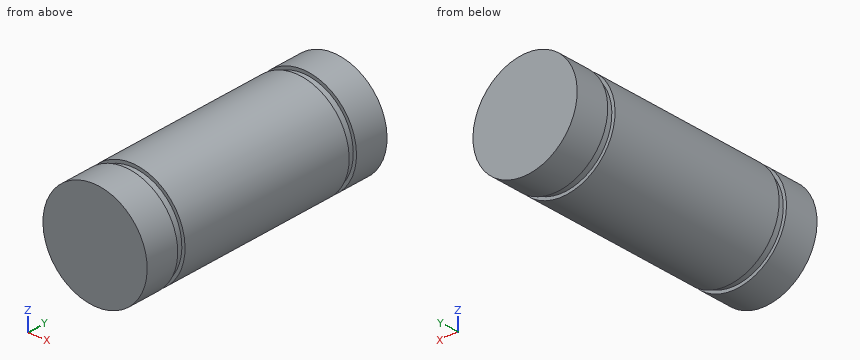
```python
from build123d import *

# Parameters (mm, degrees)
BOSS_EXTRUDE1_DEPTH      = 8.255
BOSS_EXTRUDE1_DEPTH_BACK = 8.255
SKETCH1_R                = 4.7625
SKETCH2_R                = 4.7625
BOSS_EXTRUDE2_DEPTH      = 3.81
BOSS_EXTRUDE3_START      = 3.81
SKETCH3_R                = 4.7625
BOSS_EXTRUDE3_DEPTH      = 3.81
SKETCH4_R                = 5.08
CUT_EXTRUDE1_DEPTH       = 0.7366
SKETCH5_R                = 5.08
CUT_EXTRUDE2_DEPTH       = 0.7366
SKETCH6_R                = 4.4704
BOSS_EXTRUDE4_DEPTH      = 0.7366
SKETCH7_R                = 4.4704
BOSS_EXTRUDE5_DEPTH      = 0.7366


with BuildPart() as part:
    # Sketch1 → Boss-Extrude1 (new, two sides: drawn at the far end of the back side and taken through both)
    with BuildSketch(Plane(origin=(0, 0, 0), x_dir=(1, 0, 0), z_dir=(0, 1, 0)).offset(-BOSS_EXTRUDE1_DEPTH_BACK)):
        with Locations(Location((0, 0, 0), (0, 0, 270))):
            Circle(SKETCH1_R)
    extrude(amount=BOSS_EXTRUDE1_DEPTH + BOSS_EXTRUDE1_DEPTH_BACK)

    # Sketch2 → Boss-Extrude2 (add)
    with BuildSketch(Plane(origin=(0, 8.255, 0), x_dir=(1, 0, 0), z_dir=(0, 1, 0))):
        with Locations(Location((0, 0, 0), (0, 0, 270))):
            Circle(SKETCH2_R)
    extrude(amount=BOSS_EXTRUDE2_DEPTH)

    # Sketch3 → Boss-Extrude3 (add)
    with BuildSketch(Plane(origin=(0, -8.255, 0), x_dir=(-1, 0, 0), z_dir=(0, -1, 0)).offset(BOSS_EXTRUDE3_START)):
        with Locations(Location((0, 0, 0), (0, 0, 90))):
            Circle(SKETCH3_R)
    extrude(amount=-BOSS_EXTRUDE3_DEPTH)

    # Sketch4 → Cut-Extrude1 (cut)
    with BuildSketch(Plane(origin=(0, -8.9916, 0), x_dir=(-1, 0, 0), z_dir=(0, -1, 0))):
        Circle(SKETCH4_R)
    extrude(amount=-CUT_EXTRUDE1_DEPTH, mode=Mode.SUBTRACT)


with BuildPart() as cut_extrude1_piece_1:
    # of the separate pieces the step leaves, piece 1, a body of its own (cut_extrude1_pieces)
    add(part.part.solids().sort_by_distance((0, 12.065, 4.7625))[0])

    # Sketch5 → Cut-Extrude2 (cut)
    with BuildSketch(Plane(origin=(0, 8.9916, 0), x_dir=(1, 0, 0), z_dir=(0, 1, 0))):
        Circle(SKETCH5_R)
    extrude(amount=-CUT_EXTRUDE2_DEPTH, mode=Mode.SUBTRACT)


with BuildPart() as cut_extrude1_piece_2:
    # of the separate pieces the step leaves, piece 2, a body of its own (cut_extrude1_pieces)
    add(part.part.solids().sort_by_distance((0, -12.065, -4.7625))[0])



with BuildPart() as cut_extrude2_piece_1:
    # of the separate pieces the step leaves, piece 1, a body of its own (cut_extrude2_pieces)
    add(cut_extrude1_piece_1.part.solids().sort_by_distance((0, 8.255, 4.7625))[0])


with BuildPart() as cut_extrude2_piece_2:
    # of the separate pieces the step leaves, piece 2, a body of its own (cut_extrude2_pieces)
    add(cut_extrude1_piece_1.part.solids().sort_by_distance((0, 12.065, 4.7625))[0])


with BuildPart() as cut_extrude1_piece_2_1:
    add(cut_extrude1_piece_2.part)

    add(cut_extrude2_piece_1.part)  # Boss-Extrude4 merges Cut-Extrude2 piece 1
    # Sketch6 → Boss-Extrude4 (add)
    with BuildSketch(Plane(origin=(0, -8.9916, 0), x_dir=(1, 0, 0), z_dir=(0, 1, 0))):
        with Locations(Location((0, 0, 0), (0, 0, 90))):
            Circle(SKETCH6_R)
    extrude(amount=BOSS_EXTRUDE4_DEPTH)


    add(cut_extrude2_piece_2.part)  # Boss-Extrude5 merges Cut-Extrude2 piece 2
    # Sketch7 → Boss-Extrude5 (add)
    with BuildSketch(Plane(origin=(0, 8.255, 0), x_dir=(1, 0, 0), z_dir=(0, 1, 0))):
        with Locations(Location((0, 0, 0), (0, 0, 270))):
            Circle(SKETCH7_R)
    extrude(amount=BOSS_EXTRUDE5_DEPTH)


solid = cut_extrude1_piece_2_1.part
```
Build history of the part. All positions in model axes, mm. Give positions to 0.01 mm unless a question says otherwise; leave off trailing zeros. Order: outer loops, then holes, each group sorted by start corner. A loop starts at its lowest first (then second) coordinate and runs counter-clockwise, first axis right, second up. Notation, with made-up numbers: M 59.25,34.25 L 74.25,34.25 A21 ccw 74.25,51.25 Z; hole C 21.25,88.5 d4. An arc over 180 degrees is marked long. Return JSON: item names as keys, results as strings.
Q1. Band-saw the part on B-B (z = 3). Give the cut face in (x, y) (3 decimals).
Answer list:
{"outline": "M -3.699,-12.065 L 3.699,-12.065 L 3.699,-8.992 L 3.314,-8.992 L 3.314,-8.255 L 3.699,-8.255 L 3.699,8.255 L 3.314,8.255 L 3.314,8.992 L 3.699,8.992 L 3.699,12.065 L -3.699,12.065 L -3.699,8.992 L -3.314,8.992 L -3.314,8.255 L -3.699,8.255 L -3.699,-8.255 L -3.314,-8.255 L -3.314,-8.992 L -3.699,-8.992 Z"}
Q2. Flat gauge pins, fed straight in: pin 1 (1 mm diameter, centred on y = -6, z = 1, fed in from +X); pin 2 (4 mm diameter, centred on x = -3, y = -9, fed in from -Z); pin 3 (1 mm diameter, centred on y = -1.5, z = -3.5, fed in from -X). Where does each tip first touch, or does it go through?
Answer list:
{"pin 1": "stops at x = 4.74", "pin 2": "stops at z = -4.66", "pin 3": "stops at x = -3.7"}
Q3. Band-saw the part on C-C (y = -0.75). Give the cut face in (x, z) (1 decimal), then the cut area to 3 significant figures.
Answer list:
{"outline": "C 0,0 d9.5", "area": "71.3 mm^2"}
Q4. Wall check: probe 1 along X at (y, z) = (-4, 2.75); probe 2 along Z at (x, y) = (-0.5, 1.25); probe 3 along Z at (x, y) = (-0.25, 7.25). Give the ranges that are in metal, low to high. Write a range as from..to.
Answer list:
{"probe 1": "x = -3.89..3.89", "probe 2": "z = -4.74..4.74", "probe 3": "z = -4.76..4.76"}
Q5. Band-saw the part on A-A (x = -3.75). Give the cut face in (y, z) (3 decimals).
Answer list:
{"outline": "M -12.065,-2.936 L -8.992,-2.936 L -8.992,-2.434 L -8.255,-2.434 L -8.255,-2.936 L 8.255,-2.936 L 8.255,-2.434 L 8.992,-2.434 L 8.992,-2.936 L 12.065,-2.936 L 12.065,2.936 L 8.992,2.936 L 8.992,2.434 L 8.255,2.434 L 8.255,2.936 L -8.255,2.936 L -8.255,2.434 L -8.992,2.434 L -8.992,2.936 L -12.065,2.936 Z"}
